Here's how the part is built. I have some questions about the finished solid (model axes, mm). A direction names the side the tool comes from. Coordinates: 2 decimals unless noted, no trailing zeros. Order: outer loops, then holes, each group sorted by start corner. A loop starts at its lowest first (then second) coordinate and runs counter-clockwise, first axis right, second up. Notation, with made-up numbers: (56, 46.25) -> (86, 46.25) arc R29 ccw to (86, 77.25) -> close; hole circle Ø4 at (5.5, 65.25). An arc over 180 degrees is marked (long way). One line per item, written item: value. Start each with the question number.
```python
from build123d import *

# Parameters (mm, degrees)
SKETCH_R           = 50
PAD_DEPTH          = 4
POCKET_DEPTH       = 3
POLARPATTERN_COUNT = 3


with BuildPart() as part:
    # Sketch → Pad (new body)
    with BuildSketch(Plane.XY):
        Circle(SKETCH_R)
    extrude(amount=PAD_DEPTH)

    # Sketch001 → Pocket (cut)
    with BuildSketch(Plane(origin=(0, 0, 0), x_dir=(-1, 0, 0), z_dir=(0, 0, -1))):
        with BuildLine():
            ThreePointArc((-7.987816, -45.301157), (0, -46), (7.987816, -45.301157))
            Line((7.987816, -45.301157), (8.335113, -47.270772))
            ThreePointArc((-8.335113, -47.270772), (0, -48), (8.335113, -47.270772))
            Line((-7.987816, -45.301157), (-8.335113, -47.270772))
        make_face()
    pocket = extrude(amount=-POCKET_DEPTH, mode=Mode.SUBTRACT)

    # PolarPattern: Pocket ×3 about axis
    polarpattern_axis = Axis((0, 0, 0), (0, 0, -1))
    for i in range(1, POLARPATTERN_COUNT):
        add(pocket.rotate(polarpattern_axis, i * 360 / POLARPATTERN_COUNT), mode=Mode.SUBTRACT)


solid = part.part
```
Q1. Imagine slicing it at B-B (x = -3.5). Write out the boundary of the cut face in (y, z), plus the area to 3 significant figures.
Q2. Imagine slicing it at A-A (z = 1). Write out the boundary of the cut face in (x, y).
Q3. For P1, Ø8, axis at x = -39.5, y = 25.5, coming from the -Z side; P2, Ø1.5, axis at x = 4, z = 3.5, coming from the -Y side; P3, Ø2, axis at x = 36, z = 2.5, coming from the +Y side, each with a flat end and sliding along its axis, tell me the tip position at first contact or that it passes through.
Q4. Imagine slicing it at C-C (y = 23.5). Write out the boundary of the cut face in (x, z), plus the area to 3 significant figures.
Q5. I need wall thicknesses on line 1 (X direction, y = 29, z = 0.4); line 2 (X direction, y = 20.5, z = 0.4); line 3 (Y direction, x = 0.5, z = 2.65). Which ranges of each line are inside material? Lowest first, please.
Q6. Imagine slicing it at D-D (x = 39). Write out the boundary of the cut face in (y, z).
Q7. If we mould it in two halves opening along Y, with no side actions, what happens to faces 1 (the face through (0, -46, 1)), 2 (the face through (-1, 1, 0)), 3 (the face through (47.69, 15.02, 1.97)), 4 (the face through (-39.893, 22.903, 1.479))? For each: +Y half, -Y half, draft (parallel to the pull), parting line (faces both ways), or undercut.
Q8. For faces 5 (the face through (0, -48, 1)), 6 (the face through (-1, 1, 4)), which set-ups out of +Z, -Z, +X, -X, +Y, -Y let a thin tool reach every point of the face, with its end or its side?
Completed:
1. outline: (-49.88, 0) -> (-47.87, 0) -> (-47.87, 3) -> (-45.87, 3) -> (-45.87, 0) -> (49.88, 0) -> (49.88, 4) -> (-49.88, 4) -> close
1. area: 393 mm2
2. outline: circle Ø100 at (0, 0); hole (-45.11, 16.42) -> (-43.23, 15.73) arc R46 cw to (-35.24, 29.57) -> (-36.77, 30.85) arc R48 ccw to start; hole (-8.34, -47.27) arc R48 ccw to (8.34, -47.27) -> (7.99, -45.3) arc R46 cw to (-7.99, -45.3) -> close; hole (35.24, 29.57) arc R46 cw to (43.23, 15.73) -> (45.11, 16.42) arc R48 ccw to (36.77, 30.85) -> close
3. P1: stops at z = 0
3. P2: stops at y = -49.89
3. P3: stops at y = 35.71
4. outline: (-44.13, 0) -> (-41.85, 0) -> (-41.85, 3) -> (-39.54, 3) -> (-39.54, 0) -> (39.54, 0) -> (39.54, 3) -> (41.85, 3) -> (41.85, 0) -> (44.13, 0) -> (44.13, 4) -> (-44.13, 4) -> close
4. area: 339 mm2
5. line 1: x = -40.73 to -38.25, -35.71 to 35.71, 38.25 to 40.73
5. line 2: x = -45.6 to -43.4, -41.18 to 41.18, 43.4 to 45.6
5. line 3: y = -50 to -48, -46 to 50
6. outline: (-31.29, 0) -> (24.39, 0) -> (24.39, 3) -> (27.98, 3) -> (27.98, 0) -> (31.29, 0) -> (31.29, 4) -> (-31.29, 4) -> close
7. face 1: undercut
7. face 2: draft
7. face 3: parting line
7. face 4: undercut
8. face 5: -Z
8. face 6: +Z, +X, -X, +Y, -Y
